The drawing under review shows one solid part. Ordinate dimensions are in mm from its lowest x, y, z. Round coordinates to 2 decimals unless told otherwise and drop trailing zeros. Write each loop counter-clockwise with the first axis right and the second up, starting at its lowest first coordinate (ties: lowest second). Pieces come first, ordered by that corner, then holes. Notation, with made-up numbers: (-7.75, -16) -> (21.25, -16) arc R22 cw to (21.25, 4) -> close; hole circle Ø5 at (-6.5, 60). An arc over 180 degrees is marked (long way). Answer in a Markdown table with one row per item.
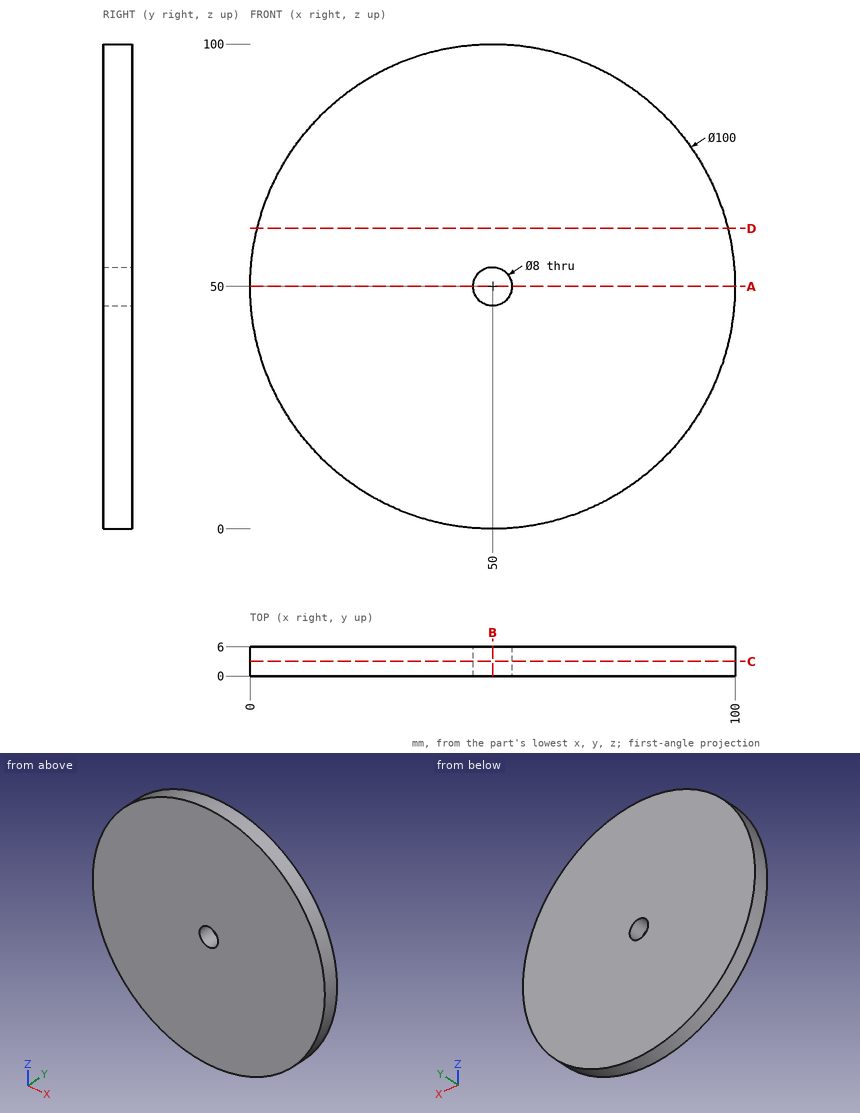
1) For line 1 (X direction, y = 3, z = 50); line 2 (Z direction, x = 53, y = 3.8), list the stretches that pass through material, from the lowest coordinate up. Write a range as [from, to].
Solved:
| item | result |
|---|---|
| line 1 | [0, 46], [54, 100] |
| line 2 | [0.09, 47.35], [52.65, 99.91] |
2) Consider section D-D on z = 62. State the section outline as (x, y) points.
Solved:
| item | result |
|---|---|
| outline | (1.46, 0) -> (98.54, 0) -> (98.54, 6) -> (1.46, 6) -> close |
3) Consider section C-C on y = 3. State the section outline as (x, z) points, then the cut area to 3 significant figures.
Solved:
| item | result |
|---|---|
| outline | circle Ø100 at (50, 50); hole circle Ø8 at (50, 50) |
| area | 7,800 mm² |
4) Clearance check with flat-ended pins moving along their axes: pin 1 Ø2 at (y, z) = (2, 52.5) entering from +X; pin 2 Ø3 at (y, z) = (1, 69) entering from -X. State where each tip first meets the part, or that it passes through.
Solved:
| item | result |
|---|---|
| pin 1 | x = 99.98 |
| pin 2 | x = 3.16 |
5) Consider section A-A on z = 50. State the section outline as (x, y) points, then the cut area to 3 significant figures.
Solved:
| item | result |
|---|---|
| outline | (0, 0) -> (46, 0) -> (46, 6) -> (0, 6) -> close; (54, 0) -> (100, 0) -> (100, 6) -> (54, 6) -> close |
| area | 552 mm² |
6) Consider section B-B on x = 50. State the section outline as (y, z) points, then the cut area to 3 significant figures.
Solved:
| item | result |
|---|---|
| outline | (0, 0) -> (6, 0) -> (6, 46) -> (0, 46) -> close; (0, 54) -> (6, 54) -> (6, 100) -> (0, 100) -> close |
| area | 552 mm² |
